The drawing under review shows one solid part. Ordinate dimensions are in mm from its lowest x, y, z. Coordinates: 2 decimals unless noted, no trailing zeros. Write each loop counter-clockwise with the first axis right and the second up, starting at its lowest first coordinate (ties: lowest second). Pieces come first, ordered by that corner, then holes.
1) To check wall thickness, follow line 1 along Z through (x, y) = (10.5, 0.6); line 2 along X through (y, z) = (0.45, 13.5); line 3 along X through (y, z) = (1.3, 2). State the ranges of each line that lie inside material, in increasing order.
2) We need section B-B on z = 6. Write out the cut boundary in (x, y).
3) We need section A-A on x = 15.75. Write out the cut boundary in (y, z).
4) We need section C-C on y = 0.5. Write out the cut boundary in (x, z).
5) Insertion check: P1, Ø0.5, axis at x = 9.5, y = 1, coming from the -Z side. The pin has a flat end and moves straight along its axis. Give the tip position at first contact, or say it passes through.
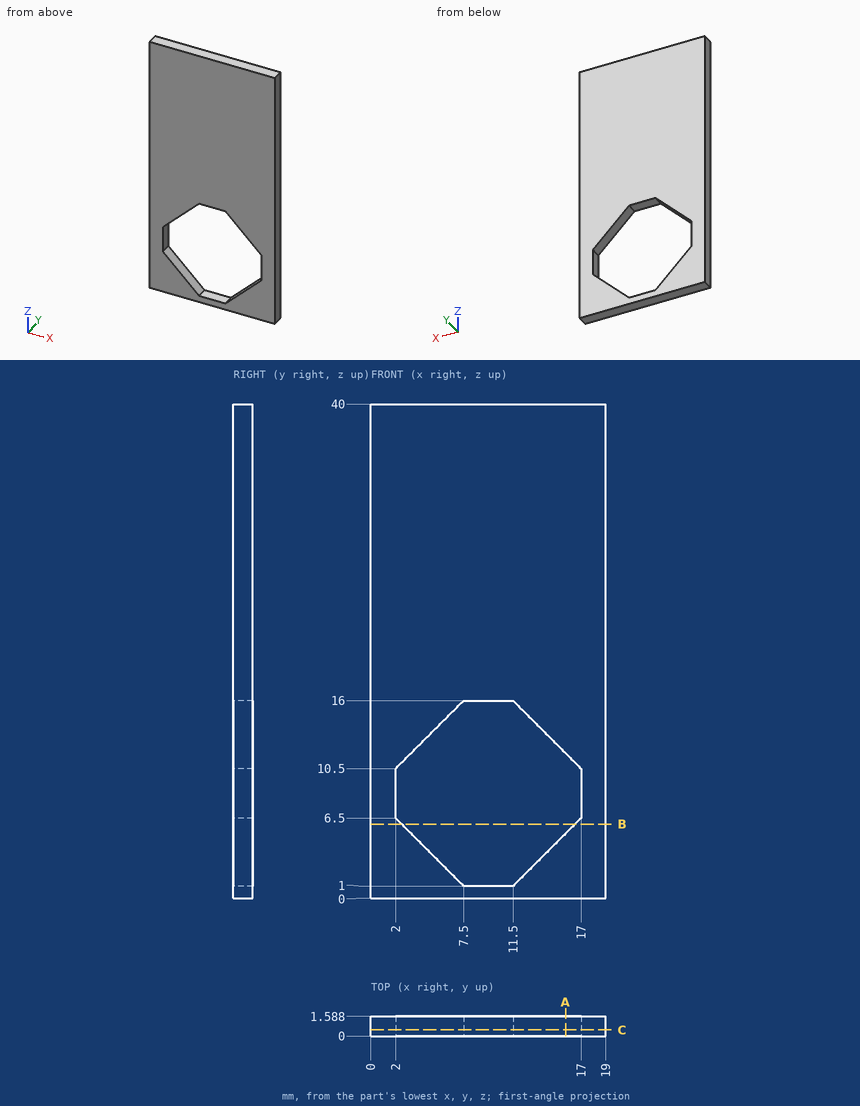
Result:
1. line 1: z = 0 to 1, 16 to 40
1. line 2: x = 0 to 5, 14 to 19
1. line 3: x = 0 to 6.5, 12.5 to 19
2. outline: (0, 0) - (2.5, 0) - (2.5, 1.59) - (0, 1.59) - close; (16.5, 0) - (19, 0) - (19, 1.59) - (16.5, 1.59) - close
3. outline: (0, 0) - (1.59, 0) - (1.59, 5.25) - (0, 5.25) - close; (0, 11.75) - (1.59, 11.75) - (1.59, 40) - (0, 40) - close
4. outline: (0, 0) - (19, 0) - (19, 40) - (0, 40) - close; hole (2, 6.5) - (7.5, 1) - (11.5, 1) - (17, 6.5) - (17, 10.5) - (11.5, 16) - (7.5, 16) - (2, 10.5) - close
5. P1: stops at z = 0
